Could you check a few things on this model? Use its own coordinates, in mm. Face numbers are marked on the shaded views. A direction names the side the tool comes from. Give positions to 0.01 mm unless a question says otherwise; leave off trailing zeros. Loops run counter-clockwise (first coordinate to the right, second up) from the corner with the lowest first, then second, coordinate; pieces in that order, holes last. Notation, with made-up numbers: (44, 31.25) -> (88, 31.25) arc R30 ccw to (88, 59.25) -> close; hole circle Ø5 at (-4.5, 67.25). An arc over 180 degrees is marked (long way). Write item = value, one per line. Start each with the question number.
1) I need wall thicknesses on probe 1 along Y at (x, z) = (0, 15.75); probe 2 along Y at (x, z) = (0, 31.5); probe 3 along Z at (x, y) = (-11, -0.5). Which ranges of each line are inside material? Lowest first, please. Write a range as from..to.
2) I want a section at B-B (z = 5). List the corners of the cut face in (x, y) for me.
3) I want a section at C-C (x = -14.5). List the corners of the cut face in (y, z) for me, and give its area (3 significant figures).
4) I want a section at A-A (y = 0). List the corners of the cut face in (x, z) for me.
5) On a 3-axis mill with a long thin cutter (end or side, diameter ignored), from which of +Z, -Z, +X, -X, +Y, -Y can I reach the whole of each face in a straight line? I mean the marked faces 5, 6 and 7. Say none if no direction works.
6) I'm going to push flat-ended pins straight in: pin 1 Ø3.5 at (y, z) = (7, -1.5) entering from +X; pin 2 Ø5 at (x, y) = (-2, 2) entering from +Z; pin 3 Ø6 at (x, z) = (-2.5, -9) entering from +Y. Where does each tip first touch, or does it pass through?
7) I want a section at D-D (y = 15). List the corners of the cut face in (x, z) for me, and give its area (3 significant figures).
8) If we mould it in two halves opening along X, with no side actions, what happens to the marked faces 1, 2, 3 and 4? For each: +X half, -X half, draft (parallel to the pull), parting line (faces both ways), or undercut.
from build123d import *

# Parameters (mm, degrees)
BOSS_EXTRUDE1_DEPTH      = 17.5
BOSS_EXTRUDE1_DEPTH_BACK = 20
BOSS_EXTRUDE2_DEPTH      = 5
BOSS_EXTRUDE2_DEPTH_BACK = 5
SKETCH4_R                = 20
BOSS_EXTRUDE3_START      = 10.5
SKETCH5_R                = 20
SKETCH5_R_2              = 12.5
BOSS_EXTRUDE3_DEPTH      = 10.5
BOSS_EXTRUDE4_START      = 20
SKETCH6_R                = 20
SKETCH6_R_2              = 6.5
BOSS_EXTRUDE4_DEPTH      = 20


with BuildPart() as part:
    # Sketch3 → Boss-Extrude1 (new, two sides: drawn at the far end of the back side and taken through both)
    with BuildSketch(Plane(origin=(0, 0, 0), x_dir=(1, 0, 0), z_dir=(0, 1, 0)).offset(-BOSS_EXTRUDE1_DEPTH_BACK)):
        with BuildLine():
            Line((-9.385342517, 4.164), (-5.617617549, 4.164))
            Line((-5.617617549, 4.164), (-3.964, 4.164))
            Line((-3.964, 4.164), (-3.964, 2.510382451))
            Line((-3.964, 2.510382451), (-3.964, 1.553617549))
            Line((-3.964, 1.553617549), (-3.964, -0.1))
            Line((-3.964, -0.1), (3.964, -0.1))
            Line((3.964, -0.1), (3.964, 1.553617549))
            Line((3.964, 1.553617549), (3.964, 2.510382451))
            Line((3.964, 2.510382451), (3.964, 4.164))
            Line((3.964, 4.164), (5.617617549, 4.164))
            Line((5.617617549, 4.164), (9.385342517, 4.164))
            ThreePointArc((9.385342517, 4.164), (9.952230024, 4.398812494), (10.187042517, 4.9657))
            Line((10.187042517, 4.9657), (10.187042517, 5.533957912))
            ThreePointArc((10.187042517, 5.533957912), (10.12601655, 5.840755675), (9.952229326, 6.100846116))
            Line((9.952229326, 6.100846116), (5.221354652, 10.831709155))
            ThreePointArc((5.221354652, 10.831709155), (3.712852366, 11.839656144), (1.933453584, 12.1936))
            Line((1.933453584, 12.1936), (-1.933453584, 12.1936))
            ThreePointArc((-1.933453584, 12.1936), (-3.712852366, 11.839656144), (-5.221354652, 10.831709155))
            Line((-5.221354652, 10.831709155), (-9.952229326, 6.100846116))
            ThreePointArc((-9.952229326, 6.100846116), (-10.12601655, 5.840755675), (-10.187042517, 5.533957912))
            Line((-10.187042517, 5.533957912), (-10.187042517, 4.9657))
            ThreePointArc((-10.187042517, 4.9657), (-9.952230024, 4.398812494), (-9.385342517, 4.164))
        make_face()
    extrude(amount=BOSS_EXTRUDE1_DEPTH + BOSS_EXTRUDE1_DEPTH_BACK)

    # Sketch4 → Boss-Extrude2 (add, two sides: drawn at the far end of the back side and taken through both)
    with BuildSketch(Plane.XY.offset(5).offset(-BOSS_EXTRUDE2_DEPTH_BACK)):
        Circle(SKETCH4_R)
    extrude(amount=BOSS_EXTRUDE2_DEPTH + BOSS_EXTRUDE2_DEPTH_BACK)

    # Sketch5 → Boss-Extrude3 (add)
    with BuildSketch(Plane.XY.offset(10).offset(BOSS_EXTRUDE3_START)):
        Circle(SKETCH5_R)
        with Locations(Location((0, 0, 0), (0, 0, 180))):
            Circle(SKETCH5_R_2, mode=Mode.SUBTRACT)
    extrude(amount=-BOSS_EXTRUDE3_DEPTH)

    # Sketch6 → Boss-Extrude4 (add)
    with BuildSketch(Plane.XY.offset(20.5).offset(BOSS_EXTRUDE4_START)):
        Circle(SKETCH6_R)
        Circle(SKETCH6_R_2, mode=Mode.SUBTRACT)
    extrude(amount=-BOSS_EXTRUDE4_DEPTH)


solid = part.part
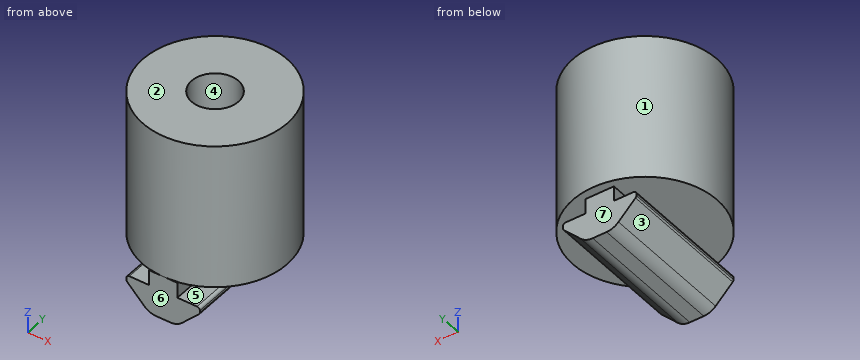
Answer list:
q1.probe_1 = -20..-12.5, 12.5..20
q1.probe_2 = -20..-6.5, 6.5..20
q1.probe_3 = 0..10, 20.5..40.5
q2.outline = circle Ø40 at (0, 0)
q3.outline = (-13.77, 0) -> (13.77, 0) -> (13.77, 40.5) -> (-13.77, 40.5) -> close
q3.area = 1,120 mm^2
q4.outline = (-20, 0) -> (-3.96, 0) -> (-3.96, -4.16) -> (-9.39, -4.16) arc R0.8 ccw to (-10.19, -4.97) -> (-10.19, -5.53) arc R0.8 ccw to (-9.95, -6.1) -> (-5.22, -10.83) arc R4.65 ccw to (-1.93, -12.19) -> (1.93, -12.19) arc R4.65 ccw to (5.22, -10.83) -> (9.95, -6.1) arc R0.8 ccw to (10.19, -5.53) -> (10.19, -4.97) arc R0.8 ccw to (9.39, -4.16) -> (3.96, -4.16) -> (3.96, 0) -> (20, 0) -> (20, 40.5) -> (6.5, 40.5) -> (6.5, 20.5) -> (12.5, 20.5) -> (12.5, 10) -> (-12.5, 10) -> (-12.5, 20.5) -> (-6.5, 20.5) -> (-6.5, 40.5) -> (-20, 40.5) -> close
q5.face_5 = +X, +Y, -Y
q5.face_6 = +Z, -Z, +X, -X, -Y
q5.face_7 = -Z, +X, -X, +Y
q6.pin_1 = 19.05
q6.pin_2 = 10
q6.pin_3 = 17.5
q7.outline = (-13.23, 0) -> (-3.96, 0) -> (-3.96, -4.16) -> (-9.39, -4.16) arc R0.8 ccw to (-10.19, -4.97) -> (-10.19, -5.53) arc R0.8 ccw to (-9.95, -6.1) -> (-5.22, -10.83) arc R4.65 ccw to (-1.93, -12.19) -> (1.93, -12.19) arc R4.65 ccw to (5.22, -10.83) -> (9.95, -6.1) arc R0.8 ccw to (10.19, -5.53) -> (10.19, -4.97) arc R0.8 ccw to (9.39, -4.16) -> (3.96, -4.16) -> (3.96, 0) -> (13.23, 0) -> (13.23, 40.5) -> (-13.23, 40.5) -> close
q7.area = 1,230 mm^2
q8.face_1 = parting line
q8.face_2 = draft
q8.face_3 = -X half
q8.face_4 = undercut
